```python
from build123d import *

# Parameters (mm, degrees)
SKETCH2_R               = 1
BOSS_EXTRUDE1_DEPTH     = 16
SKETCH3_R               = 0.95
BOSS_EXTRUDE2_DEPTH     = 2.5
CUT_EXTRUDE1_DEPTH      = 17.385969608
CUT_EXTRUDE1_DEPTH_BACK = 17.385969608
SKETCH4_W               = 6.5
SKETCH4_H               = 2.5
FILLET1_R               = 1
FILLET2_R               = 0.2
FILLET3_R               = 0.2
FILLET4_R               = 0.2


with BuildPart() as part:
    # Sketch2 → Boss-Extrude1 (new body)
    with BuildSketch(Plane(origin=(0, 0, 0), x_dir=(0, 0, -1), z_dir=(1, 0, 0))):
        Circle(SKETCH2_R)
    extrude(amount=BOSS_EXTRUDE1_DEPTH)

    # Sketch3 → Boss-Extrude2 (add, symmetric)
    with BuildSketch(Plane.XY):
        with BuildLine():
            Line((0, -2.125), (0, 2.125))
            Line((0, 2.125), (-5.06876613, 2.493422203))
            ThreePointArc((-5.06876613, 2.493422203), (-7.75, 0), (-5.06876613, -2.493422203))
            Line((-5.06876613, -2.493422203), (0, -2.125))
        make_face()
        with Locations((-5.25, 0)):
            Circle(SKETCH3_R, mode=Mode.SUBTRACT)
    extrude(amount=BOSS_EXTRUDE2_DEPTH, both=True)

    # Sketch4 → Cut-Extrude1 (cut, two sides: drawn at the far end of the back side and taken through both)
    with BuildSketch(Plane(origin=(0, 0, 0), x_dir=(1, 0, 0), z_dir=(0, 1, 0)).offset(-CUT_EXTRUDE1_DEPTH_BACK)):
        with Locations((-4.5, 0)):
            Rectangle(SKETCH4_W, SKETCH4_H)
    extrude(amount=CUT_EXTRUDE1_DEPTH + CUT_EXTRUDE1_DEPTH_BACK, mode=Mode.SUBTRACT)

    # Fillet1
    fillet1_edges = [part.edges().sort_by_distance(p)[0] for p in [
        (0, 0, 2.5),
        (0, 0, -2.5),
    ]]
    fillet(fillet1_edges, radius=FILLET1_R)

    # Fillet2
    fillet2_edges = [part.edges().sort_by_distance(p)[0] for p in [
        (0, 2.125, 0),
        (0, -2.125, 0),
        (-3.034383065, 2.345553497, 2.5),
        (-3.034383065, 2.345553497, -2.5),
        (-0.293359104, 2.146322745, 2.20757236),
        (-0.293359104, 2.146322745, -2.20757236),
        (-0.293359104, -2.146322745, 2.20757236),
        (-0.293359104, -2.146322745, -2.20757236),
        (-3.034383065, -2.345553497, 2.5),
        (-7.75, 0, 2.5),
        (-3.034383065, -2.345553497, -2.5),
        (-7.75, 0, -2.5),
    ]]
    fillet(fillet2_edges, radius=FILLET2_R)

    # Fillet3
    fillet3_edges = [part.edges().sort_by_distance(p)[0] for p in [
        (-7.75, 0, -1.25),
        (-3.159383065, 2.354639096, -1.25),
        (-3.159383065, -2.354639096, -1.25),
    ]]
    fillet(fillet3_edges, radius=FILLET3_R)

    # Fillet4
    fillet4_edges = [part.edges().sort_by_distance(p)[0] for p in [
        (-7.75, 0, 1.25),
        (-3.159383065, -2.354639096, 1.25),
        (-3.159383065, 2.354639096, 1.25),
    ]]
    fillet(fillet4_edges, radius=FILLET4_R)


solid = part.part
```
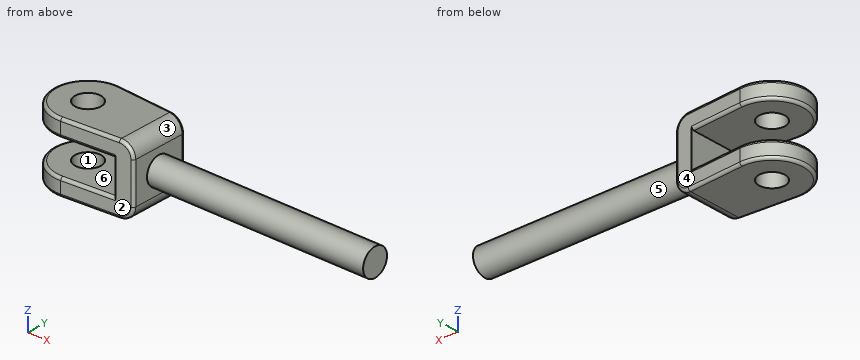
Check sheet for the modelled part. Datum: model origin and axes. Units: mm. Face numbers are marked on the shaded views. A direction names the side the tool comes from. Coordinates: 2 decimals unless noted, no trailing zeros. Order: outer loops, then holes, each group sorted by start corner. A loop starts at its lowest first (then second) coordinate and runs counter-clockwise, first axis right, second up. Notation, with made-up numbers: (31.5, -38) -> (82.5, -38) arc R21 ccw to (82.5, -34) -> close; hole circle Ø5 at (-10.75, 88). An arc over 180 degrees is marked (long way). Write item = value, one per line. Start each with the question number.
1) Access from +Z, -Z, +X, -X, +Y, -Y to the whole of each face (thin tool, end or side, straight path). Record for the marked faces 4, 5 and 6.
2) Material ranges on L1, parallel to Z at x = -6.25, y = 0.45; L2, parallel to Y at x = -5.25, z = 2.15; L3, parallel to X at y = -1.25, z = -0.6, recorded low to high.
3) Cross-section at B-B (z = 0). Enter the section's corners in (x, y), then the cut area to 3 significant figures.
4) Mould release check, pull along Y, two halves, no side actions. Record for the marked faces 1, 2 and 3: +Y half, -Y half, draft (parallel to the pull), parting line (faces both ways), or undercut.
5) Cross-section at A-A (y = 0). Enter the section's corners in (x, z), then the cut area to 3 significant figures.
6) Cross-section at C-C (x = 11). Enter the section's corners in (y, z).
7) Go/stop test with flat-tipped pins: P1, Ø1, axis at x = 3, y = -0.5, coming from the +Z side; P2, Ø3, axis at x = -5.25, y = 0, coming from the +Z side; P3, Ø1.5, axis at x = 2.5, y = -2, coming from the +Z side; P4, Ø0.9, axis at y = 0.5, z = 0, coming from the -X side. Record where each tip stops, or that it passes through.
Ans:
q1.face_4 = +Z, -Z, +X, +Y
q1.face_5 = +X
q1.face_6 = -X, +Y, -Y
q2.L1 = -2.5 to -1.25, 1.25 to 2.5
q2.L2 = -2.5 to -0.95, 0.95 to 2.5
q2.L3 = -1.25 to 0
q3.outline = (-1.25, -2.22) -> (-0.19, -2.14) arc R0.2 ccw to (0, -1.94) -> (0, -1) -> (16, -1) -> (16, 1) -> (0, 1) -> (0, 1.94) arc R0.2 ccw to (-0.19, 2.14) -> (-1.25, 2.22) -> close
q3.area = 37.4 mm²
q4.face_1 = undercut
q4.face_2 = -Y half
q4.face_3 = draft
q5.outline = (-7.75, -2.3) arc R0.2 ccw to (-7.55, -2.5) -> (-6.2, -2.5) -> (-6.2, -1.25) -> (-7.55, -1.25) arc R0.2 ccw to (-7.75, -1.45) -> close; (-7.75, 1.45) arc R0.2 ccw to (-7.55, 1.25) -> (-6.2, 1.25) -> (-6.2, 2.5) -> (-7.55, 2.5) arc R0.2 ccw to (-7.75, 2.3) -> close; (-4.3, -2.5) -> (-1, -2.5) arc R1 ccw to (0, -1.5) -> (0, -1) -> (16, -1) -> (16, 1) -> (0, 1) -> (0, 1.5) arc R1 ccw to (-1, 2.5) -> (-4.3, 2.5) -> (-4.3, 1.25) -> (-1.25, 1.25) -> (-1.25, -1.25) -> (-4.3, -1.25) -> close
q5.area = 49.3 mm²
q6.outline = circle Ø2 at (0, 0)
q7.P1 = 1
q7.P2 = 2.5
q7.P3 = through
q7.P4 = -1.25
